Model file for the job. Use its own axes, mm. Face numbers are marked on the shaded views. A direction names the side the tool comes from. Coordinates: 2 decimals unless noted, no trailing zeros. Loops run counter-clockwise (first coordinate to the right, second up) from the corner with the lowest first, then second, coordinate; pieces in that order, holes last.
from build123d import *

# Parameters (mm, degrees)
F0_R     = 25.603668
F1_DEPTH = 25.4


with BuildPart() as f1:
    # F0 (on Front) → F1 (new body)
    with BuildSketch(Plane.XZ):
        with BuildLine():
            Line((-75.622357, 0), (-76.396644, -45.941226))
            Line((-76.396644, -45.941226), (76.65474, -45.941226))
            Line((76.65474, -45.941226), (76.396652, 0))
            Line((76.396652, 0), (42.844061, 0))
            ThreePointArc((42.844061, 0), (0.774289, 41.016271), (-41.295484, 0))
            Line((-41.295484, 0), (-75.622357, 0))
        make_face()
        Circle(F0_R, mode=Mode.SUBTRACT)
    extrude(amount=F1_DEPTH)


solid = f1.part
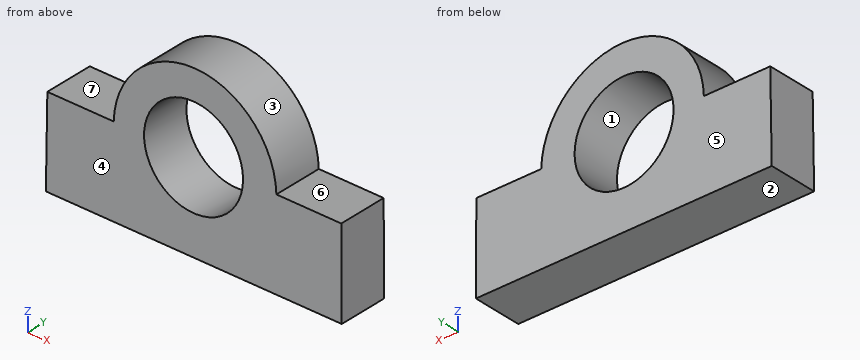
Q1. Slice it at A-A (z = 14). List the corners of the cut face in (x, y), and give its area (3 significant figures).
Answers:
outline: (-38.52, -25.4) - (-21.44, -25.4) - (-21.44, 0) - (-38.52, 0) - close; (21.44, -25.4) - (40.07, -25.4) - (40.07, 0) - (21.44, 0) - close
area: 907 mm2
Q2. Which spindle directions (+Z, -Z, +X, -X, +Y, -Y) get a long thin tool onto all of the face, cutting with end or side? Do the marked faces 5, 6 and 7. Say none if no direction does.
Answers:
face 5: +Z, -Z, +X, -X, +Y
face 6: +Z, +X, +Y, -Y
face 7: +Z, -X, +Y, -Y
Q3. Slice it at C-C (y = -23). List the corners of the cut face in (x, z), and give its area (3 significant figures).
Answers:
outline: (-76.4, -45.94) - (76.65, -45.94) - (76.4, 0) - (42.84, 0) arc R42.08 ccw to (-41.3, 0) - (-75.62, 0) - close; hole circle Ø51.21 at (0, 0)
area: 7,640 mm2
Q4. Slice it at D-D (x = -64.5). List the corners of the cut face in (y, z).
Answers:
outline: (-25.4, -45.94) - (0, -45.94) - (0, 0) - (-25.4, 0) - close
Q5. Flat gauge pins, fed straight in: P1, Ø3, axis at y = -9, z = 2.5, coming from the +X side; P2, Ø2, axis at x = -59.5, y = -6, coming from the +Z side; P3, Ø5, axis at y = -11, z = -34.5, coming from the +X side. Where does each tip first touch, or does it go through?
Answers:
P1: stops at x = 42.81
P2: stops at z = 0
P3: stops at x = 76.6
Q6. Drill centre lines: line 1 (Z direction, x = 0, y = -15.25); line 2 (X direction, y = -5.5, z = 16); line 3 (Z direction, x = 49, y = -22). Where is each one in solid material? Low to high.
Answers:
line 1: z = -45.94 to -25.6, 25.6 to 41.01
line 2: x = -37.69 to -19.99, 19.99 to 39.24
line 3: z = -45.94 to 0
Q7. Slice it at B-B (x = 15). List the corners of the cut face in (y, z), and give its area (3 significant figures).
Answers:
outline: (-25.4, -45.94) - (0, -45.94) - (0, -20.75) - (-25.4, -20.75) - close; (-25.4, 20.75) - (0, 20.75) - (0, 38.54) - (-25.4, 38.54) - close
area: 1,090 mm2
Q8. Mould opens along Z. For the marked faces 1, 2, 3 and 4 say: +Z half, -Z half, draft (parallel to the pull), parting line (faces both ways), or undercut.
Answers:
face 1: undercut
face 2: -Z half
face 3: +Z half
face 4: draft
